Verification items for the finished model (mm, model axes). Face numbers are marked on the shaded views. A direction names the side the tool comes from. Give positions to 0.01 mm unless a question says otherwise; leave off trailing zeros. Write each loop counter-clockwise with the first axis right and the second up, starting at its lowest first coordinate (ties: lowest second). Pieces come first, ordered by that corner, then holes. Notation, with made-up numbers: (26.5, -16) -> (47.5, -16) arc R28 ccw to (47.5, 3) -> close; hole circle Ø8 at (40.25, 37). An arc over 180 degrees is marked (long way). Answer as CSV lines item,"result".
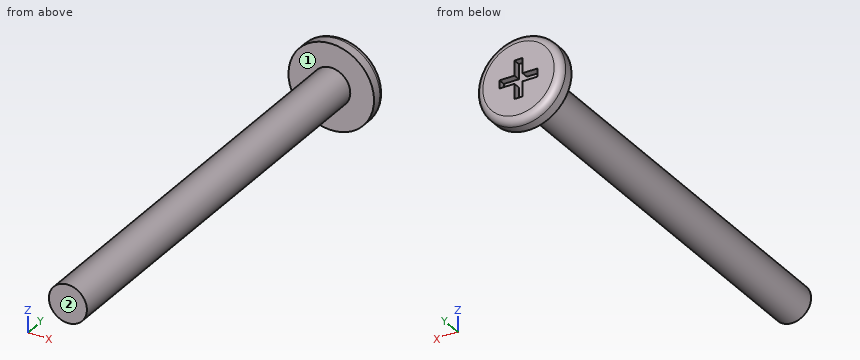
```python
from build123d import *

# Parameters (mm, degrees)
SKETCH3_R           = 2
BOSS_EXTRUDE1_DEPTH = 45
SKETCH4_R           = 4.5
BOSS_EXTRUDE2_DEPTH = 1.75
FILLET3_R           = 0.75
CUT_EXTRUDE4_DEPTH  = 0.75


with BuildPart() as part:
    # Sketch3 → Boss-Extrude1 (new body)
    with BuildSketch(Plane(origin=(0, 0, 0), x_dir=(1, 0, 0), z_dir=(0, 1, 0))):
        with Locations(Location((0, 0, 0), (0, 0, 90))):
            Circle(SKETCH3_R)
    extrude(amount=BOSS_EXTRUDE1_DEPTH)

    # Sketch4 → Boss-Extrude2 (add)
    with BuildSketch(Plane(origin=(0, 45, 0), x_dir=(1, 0, 0), z_dir=(0, 1, 0))):
        with Locations(Location((0, 0, 0), (0, 0, 270))):
            Circle(SKETCH4_R)
    extrude(amount=BOSS_EXTRUDE2_DEPTH)

    # Fillet3
    fillet3_edges = [part.edges().sort_by_distance(p)[0] for p in [
        (0, 46.75, -4.5),
    ]]
    fillet(fillet3_edges, radius=FILLET3_R)

    # Sketch6 → Cut-Extrude4 (cut)
    with BuildSketch(Plane(origin=(0, 46.75, 0), x_dir=(1, 0, 0), z_dir=(0, 1, 0))):
        Polygon((0.425, 0.425), (2, 0.425), (2, -0.425), (0.425, -0.425), (0.425, -2), (-0.425, -2), (-0.425, -0.425), (-2, -0.425), (-2, 0.425), (-0.425, 0.425), (-0.425, 2), (0.425, 2), align=None)
    extrude(amount=-CUT_EXTRUDE4_DEPTH, mode=Mode.SUBTRACT)


solid = part.part
```
1) Depth check by flat-ended pin: pin 1 (1.5 mm diameter, centred on x = -3, z = 1, fed in from -Y); pin 2 (1 mm diameter, centred on y = 20, z = 0, fed in from -X); pin 3 (0.6 mm diameter, centred on y = 46.5, z = 0, fed in from -X). Enter the tip coordinate at first touch or a pass-through.
Reported:
pin 1,"y = 45"
pin 2,"x = -2"
pin 3,"x = -4.47"
2) Scan lines: line 1 along Y through (x, z) = (3, 0.75); line 2 along Y through (x, z) = (-0.75, 0.25); line 3 along Z through (x, y) = (0.5, 31). Record each from-to range of solid material in increasing order.
Reported:
line 1,"45 to 46.75"
line 2,"0 to 46"
line 3,"-1.94 to 1.94"
3) Section check A-A (x = 0). Record the boundary of the cut face in (y, z), and give its area (3 significant figures).
Reported:
outline,"(0, -2) -> (45, -2) -> (45, -4.5) -> (46, -4.5) arc R0.75 ccw to (46.75, -3.75) -> (46.75, -2) -> (46, -2) -> (46, 2) -> (46.75, 2) -> (46.75, 3.75) arc R0.75 ccw to (46, 4.5) -> (45, 4.5) -> (45, 2) -> (0, 2) -> close"
area,"193 mm²"
4) Section check C-C (y = 18). Record the boundary of the cut face in (x, z).
Reported:
outline,"circle Ø4 at (0, 0)"
5) Section check B-B (z = 0). Record the boundary of the cut face in (x, y).
Reported:
outline,"(-4.5, 45) -> (-2, 45) -> (-2, 0) -> (2, 0) -> (2, 45) -> (4.5, 45) -> (4.5, 46) arc R0.75 ccw to (3.75, 46.75) -> (2, 46.75) -> (2, 46) -> (-2, 46) -> (-2, 46.75) -> (-3.75, 46.75) arc R0.75 ccw to (-4.5, 46) -> close"
6) Tool access check on the marked faces 1 and 2. Record the directions out of +Z, -Z, +X, -X, +Y, -Y that give a thin tool (end or side, any length) a straight path to the whole face; none if there is none.
Reported:
face 1,"-Y"
face 2,"+Z, -Z, +X, -X, -Y"
